Can you work these out from the drawing? Everything is in mm from the part's minimum corner. A direction names the side the tool comes from. Round coordinates to 2 decimals unless told otherwise and drop trailing zeros. Order: outer loops, then holes, each group sorted by start corner. A loop starts at its lowest first (then second) coordinate and runs counter-clockwise, first axis right, second up. Notation, with made-up numbers: M 32,-29.5 L 57,-29.5 A26 ccw 57,0.5 Z; hole C 73.5,68 d1. An arc over 180 degrees is marked long. Write each question's results on one line, items separated by ' | '. Start each with the question number.
1. We'd pull the mould along X, two halves only. Please class the marked faces 5, 6 and 7: released by +X, released by -X, zero draft, split by the parting line, or undercut.
2. Suppose I cut it at C-C on x = 34.1. Write out the boundary of the cut face in (y, z), and give its area (3 significant figures).
3. For the marked faces 1, 2, 3 and 4, which set-ups out of +Z, -Z, +X, -X, +Y, -Y let a thin tool reach every point of the face, with its end or its side?
4. Please list where these lines run through material, in increasing order: L1, parallel to Y at x = 34.1, z = 1.75; L2, parallel to X at y = 39, z = 3; L3, parallel to X at y = 24.5, z = 33.
5. Suppose I cut it at D-D on y = 34. Write out the boundary of the cut face in (x, z), and give its area (3 significant figures).
6. Suppose I cut it at A-A on y = 10.9. Write out the boundary of the cut face in (x, z).
7. I'm going to push flat-ended pins straight in: pin 1 (4.5 mm diameter, centred on x = 34.1, y = 10.9, fed in from +Z); pin 2 (1 mm diameter, centred on x = 43, z = 18, fed in from -Y); pin 3 (14 mm diameter, centred on y = 40, z = 21.5, fed in from -X). Where does each tip first touch, or does it pass through?
8. Suppose I cut it at B-B on z = 7. Write out the boundary of the cut face in (x, y), and give its area (3 significant figures).
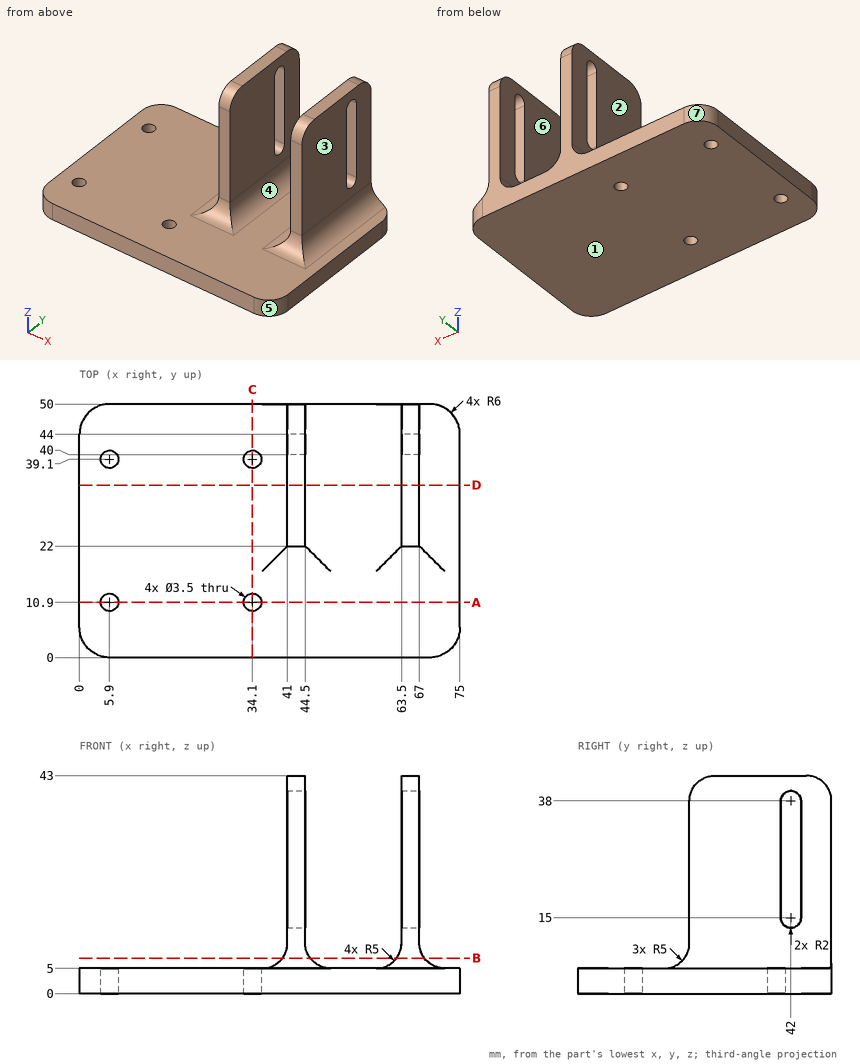
Filled sheet:
1) face 5: released by +X | face 6: undercut | face 7: released by -X
2) outline: M 0,0 L 9.15,0 L 9.15,5 L 0,5 Z; M 12.65,0 L 37.35,0 L 37.35,5 L 12.65,5 Z; M 40.85,0 L 50,0 L 50,5 L 40.85,5 Z | area: 215 mm^2
3) face 1: -Z, +X, -X, +Y, -Y | face 2: +Z, -X, +Y, -Y | face 3: +Z, +X, +Y, -Y | face 4: +Z, +Y, -Y
4) L1: y = 0 to 9.15, 12.65 to 37.35, 40.85 to 50 | L2: x = 0 to 4.15, 7.65 to 32.35, 35.85 to 75 | L3: x = 41 to 44.5, 63.5 to 67
5) outline: M 0,0 L 75,0 L 75,5 L 72,5 A5 cw 67,10 L 67,43 L 63.5,43 L 63.5,10 A5 cw 58.5,5 L 49.5,5 A5 cw 44.5,10 L 44.5,43 L 41,43 L 41,10 A5 cw 36,5 L 0,5 Z | area: 662 mm^2
6) outline: M 0,0 L 4.15,0 L 4.15,5 L 0,5 Z; M 7.65,0 L 32.35,0 L 32.35,5 L 7.65,5 Z; M 35.85,0 L 75,0 L 75,5 L 35.85,5 Z
7) pin 1: stops at z = 5 | pin 2: stops at y = 22 | pin 3: stops at x = 41
8) outline: M 40,21 L 45.5,21 L 45.5,50 L 40,50 Z; M 62.5,21 L 68,21 L 68,50 L 62.5,50 Z | area: 319 mm^2
